from build123d import *

# Parameters (mm, degrees)
SKETCH1_R          = 2
EXTRUDE1_DEPTH     = 17.3
SKETCH6_R          = 3.5
EXTRUDE2_DEPTH     = 1.3
CUT_EXTRUDE1_DEPTH = 0.975
SKETCH8_R          = 1.443375673
CUT_EXTRUDE2_DEPTH = 0.975
CUT_EXTRUDE2_TAPER = 45
CHAMFER1_SIZE      = 0.35


with BuildPart() as part:
    # Sketch1 → Extrude1 (new body)
    with BuildSketch(Plane.XY):
        Circle(SKETCH1_R)
    extrude(amount=EXTRUDE1_DEPTH)

    # Sketch4 → Cut-Revolve1 (revolve, cut)
    with BuildSketch(Plane(origin=(0, 0, 0), x_dir=(0, 0, -1), z_dir=(1, 0, 0))):
        Polygon((-16.809854723, 2), (-17.3, 1.3), (-17.3, 2), align=None)
    revolve(axis=Axis((0, 0, 0), (0, 0, 1)), mode=Mode.SUBTRACT)

    # Sketch6 → Extrude2 (add)
    with BuildSketch(Plane.XY):
        Circle(SKETCH6_R)
    extrude(amount=EXTRUDE2_DEPTH)

    # Sketch7 → Cut-Extrude1 (cut)
    with BuildSketch(Plane.XY):
        Polygon((0, 1.443375673), (-1.25, 0.721687836), (-1.25, -0.721687836), (0, -1.443375673), (1.25, -0.721687836), (1.25, 0.721687836), align=None)
    extrude(amount=CUT_EXTRUDE1_DEPTH, mode=Mode.SUBTRACT)

    # Sketch8 → Cut-Extrude2 (cut)
    with BuildSketch(Plane.XY):
        Circle(SKETCH8_R)
    extrude(amount=CUT_EXTRUDE2_DEPTH, taper=CUT_EXTRUDE2_TAPER, mode=Mode.SUBTRACT)

    # Chamfer1
    chamfer1_edges = [part.edges().sort_by_distance(p)[0] for p in [
        (-3.5, 0, 1.3),
        (-3.5, 0, 0),
    ]]
    chamfer(chamfer1_edges, length=CHAMFER1_SIZE)


solid = part.part
Check sheet for the modelled part. Datum: model origin and axes. Units: mm. A direction names the side the tool comes from. Round coordinates to 2 decimals unless told otherwise and drop trailing zeros. Order: outer loops, then holes, each group sorted by start corner. A loop starts at its lowest first (then second) coordinate and runs counter-clockwise, first axis right, second up.
Q1. Depth check by flat-ended pin: P1, Ø3, axis at x = -0.5, y = 0.5, coming from the -Z side; P2, Ø1, axis at y = -0.5, z = 7, coming from the +X side; P3, Ø4, axis at y = 2, z = 2.5, coming from the +X side. Enter the tip coordinate at first touch or a pass-through.
Filled sheet:
P1: stops at z = 0
P2: stops at x = 2
P3: stops at x = 3.42
Q2. Draft check along X on faces 1 (the face through (3.233, -1.341, 0.646)), 2 (the face through (1.25, 0, 0.6)), 3 (the face through (1, -2, 1.3)). Enter one of: pulls with the +X half, pulls with the -X half, needs draft (parallel to the pull), parting line crosses it, or undercut.
Filled sheet:
face 1: parting line crosses it
face 2: undercut
face 3: needs draft
Q3. Set-up check for faces 4 (the face through (1.847, -0.766, 8.946)), 5 (the face through (0, 0, 17.3)), 6 (the face through (0, 0, 0.975)): record each of +Z, -Z, +X, -X, +Y, -Y from which the full face is reachable in a straight line by a thin tool's end or side.
Filled sheet:
face 4: +Z
face 5: +Z, +X, -X, +Y, -Y
face 6: -Z
Q4. Scan lines: L1, parallel to Z at x = 2.5, y = 0.25; L2, parallel to Y at x = 1, z = 8; L3, parallel to Y at x = 1.5, z = 8.25. Record each from-to range of solid material in increasing order.
Filled sheet:
L1: z = 0 to 1.3
L2: y = -1.73 to 1.73
L3: y = -1.32 to 1.32
Q5. Cross-section at A-A, the plane y = 0. Enter the section's corners in (x, z) (3 decimals), plus the area to 3 significant figures.
Filled sheet:
outline: (-3.5, 0.35) - (-3.15, 0) - (-1.443, 0) - (-1.25, 0.193) - (-1.25, 0.975) - (1.25, 0.975) - (1.25, 0.193) - (1.443, 0) - (3.15, 0) - (3.5, 0.35) - (3.5, 0.95) - (3.15, 1.3) - (2, 1.3) - (2, 16.81) - (1.3, 17.3) - (-1.3, 17.3) - (-2, 16.81) - (-2, 1.3) - (-3.15, 1.3) - (-3.5, 0.95) - close
area: 70.0 mm2
Q6. Cross-section at B-B, the plane z = 15.25. Enter the section's corners in (x, y), plus the area to 3 significant figures.
Filled sheet:
outline: circle Ø4 at (0, 0)
area: 12.6 mm2
